from build123d import *

# Parameters (mm, degrees)
F2_R     = 15.5575
F3_DEPTH = 1.6891
F1_R     = 14.29385
F4_DEPTH = 7.8994
F5_DEPTH = 25.4


with BuildPart() as f3:
    # F2 (on Top) → F3 (new body)
    with BuildSketch(Plane.XY):
        Circle(F2_R)
    extrude(amount=F3_DEPTH)

    # F1 (on Top) → F4 (join)
    with BuildSketch(Plane.XY):
        Circle(F1_R)
    extrude(amount=F4_DEPTH)

    # F0 (on Top) → F5 (cut)
    with BuildSketch(Plane.XY):
        Polygon((1.999529, -7.054447), (7.109095, -1.79558), (5.109565, 5.258866), (-1.999529, 7.054447), (-7.109095, 1.79558), (-5.109565, -5.258866), align=None)
    extrude(amount=F5_DEPTH, mode=Mode.SUBTRACT)


solid = f3.part
Can you work these out from the model? Positions are in its coordinate system, mm. A direction names the side the tool comes from. Coordinates: 2 decimals unless noted, no trailing zeros. Write each loop counter-clockwise with the first axis right and the second up, starting at its lowest first coordinate (ties: lowest second). Pieces come first, ordered by that corner, then holes. Notation, with made-up numbers: M -11.5,31 L 9.5,31 A25 ccw 9.5,44 Z; hole C 54,3 d10. An arc over 180 degrees is marked long. Use one line per item in the form item = value.
Q1. If we section it at D-D (x = 11): Write out the boundary of the cut face in (y, z).
Model answer:
outline = M -11,0 L 11,0 L 11,1.69 L 9.13,1.69 L 9.13,7.9 L -9.13,7.9 L -9.13,1.69 L -11,1.69 Z
Q2. If we section it at B-B (x = 0): Write out the boundary of the cut face in (y, z).
Model answer:
outline = M -15.56,0 L -6.55,0 L -6.55,7.9 L -14.29,7.9 L -14.29,1.69 L -15.56,1.69 Z; M 6.55,0 L 15.56,0 L 15.56,1.69 L 14.29,1.69 L 14.29,7.9 L 6.55,7.9 Z
Q3. If we section it at A-A (z = 7.25): Write out the boundary of the cut face in (x, y).
Model answer:
outline = C 0,0 d28.59; hole M -7.11,1.8 L -5.11,-5.26 L 2,-7.05 L 7.11,-1.8 L 5.11,5.26 L -2,7.05 Z
Q4. If we section it at C-C (y = 0): Write out the boundary of the cut face in (x, z), then the cut area to 3 significant figures.
Model answer:
outline = M -15.56,0 L -6.6,0 L -6.6,7.9 L -14.29,7.9 L -14.29,1.69 L -15.56,1.69 Z; M 6.6,0 L 15.56,0 L 15.56,1.69 L 14.29,1.69 L 14.29,7.9 L 6.6,7.9 Z
area = 126 mm^2
Q5. We'd pull the mould along Y, two halves only. Please class faces 1 (the cylindrical face through (-1.861, 14.172, 4.751)), 2 (the flat face through (1.605, 6.144, 3.894)), 3 (the flat face through (7, 0, 0)): +Y half, -Y half, draft (parallel to the pull), parting line (faces both ways), or undercut.
Model answer:
face_1 = parting line
face_2 = undercut
face_3 = draft
Q6. For faces 4 (the flat face through (7, -13, 1.689)), 5 (the flat face through (6.2, -3, 7.899)), 6 (the flat face through (-6.123, -1.682, 3.894)), which set-ups out of +Z, -Z, +X, -X, +Y, -Y let a thin tool reach every point of the face, with its end or its side?
Model answer:
face_4 = +Z
face_5 = +Z, +X, -X, +Y, -Y
face_6 = +Z, -Z
Q7. I need wall thicknesses on line 1 along Y through (x, z) = (4, 5); line 2 along Z through (x, y) = (13, -6.5); line 3 along Y through (x, z) = (5, 4.5). Which ranges of each line are inside material? Lowest first, please. Write a range as from..to.
Model answer:
line_1 = -13.72..-5, 5.54..13.72
line_2 = 0..1.69
line_3 = -13.39..-3.97, 5.29..13.39
Q8. For P1, Ø1, axis at y = -4.5, z = 2, coming from the -X side; P2, Ø2, axis at y = -9, z = 3, coming from the +X side, each with a flat end and sliding along its axis, tell me the tip position at first contact or that it passes through.
Model answer:
P1 = -15.01
P2 = 11.85
